from build123d import *

# Parameters (mm, degrees)
SKETCH1_W           = 10
SKETCH1_H           = 10
SKETCH1_R           = 2.25
BOSS_EXTRUDE1_DEPTH = 5
CUT_EXTRUDE1_START  = -1.75
CUT_EXTRUDE1_DEPTH  = 1.55
FILLET1_R           = 5


with BuildPart() as part:
    # Sketch1 → Boss-Extrude1 (new body)
    with BuildSketch(Plane(origin=(0, 0, 0), x_dir=(1, 0, 0), z_dir=(0, 1, 0))):
        Rectangle(SKETCH1_W, SKETCH1_H)
        with Locations(Location((0, 0, 0), (0, 0, 270))):
            Circle(SKETCH1_R, mode=Mode.SUBTRACT)
    extrude(amount=BOSS_EXTRUDE1_DEPTH)

    # Sketch2 → Cut-Extrude1 (cut)
    with BuildSketch(Plane(origin=(0, 5, 0), x_dir=(1, 0, 0), z_dir=(0, 1, 0)).offset(CUT_EXTRUDE1_START)):
        Polygon((-3, 5), (-5, 5), (-5, -5), (5, -5), (5, -3), (-3, -3), align=None)
    extrude(amount=-CUT_EXTRUDE1_DEPTH, mode=Mode.SUBTRACT)

    # Fillet1
    fillet1_edges = [part.edges().sort_by_distance(p)[0] for p in [
        (5, 2.5, -5),
    ]]
    fillet(fillet1_edges, radius=FILLET1_R)


solid = part.part
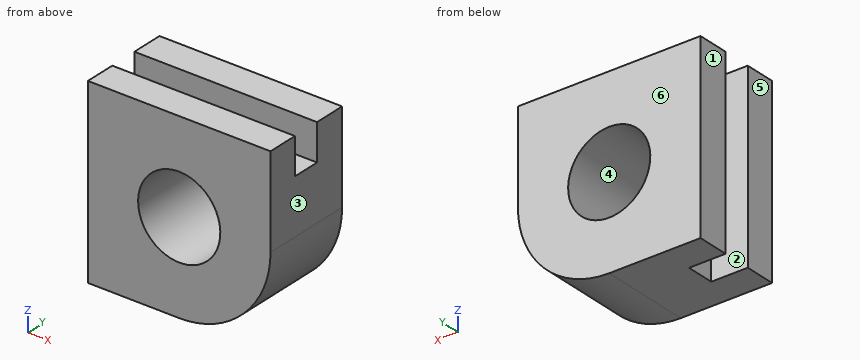
Can you work these out from the model? Positions are in its coordinate system, mm. Face numbers are marked on the shaded views. A direction names the side the tool comes from. Round coordinates to 2 decimals unless told otherwise and drop trailing zeros. Write each loop counter-clockwise with the first axis right and the second up, starting at its lowest first coordinate (ties: lowest second). Pieces come first, ordered by that corner, then holes. Notation, with made-up numbers: (34.5, 61) -> (80.5, 61) arc R24 cw to (80.5, 77) -> close; hole circle Ø11 at (80, -29). An arc over 180 degrees is marked (long way). Use one line per item in the form item = value. Start each with the question number.
Q1. Imagine slicing it at C-C (z = 2.75). Please give me the cut outline in (x, y), then the cut area to 3 significant figures.
Q2. Imagine slicing it at A-A (x = -4). Please give me the cut outline in (y, z), then the cut area to 3 significant figures.
Q3. Imagine slicing it at D-D (z = 0.5). Please give me the cut outline in (x, y).
Q4. If I drill on probe 1 along X at (y, z) = (3.05, 0); probe 2 along X at (y, z) = (0.95, 0); probe 3 along Y at (x, z) = (2.75, 3.5), over which ranges is the centre line in solid material (lowest first)? Write a range as [from, to].
Q5. We'd pull the mould along X, two halves only. Please class the marked faces 3, 4, 5 and 6: +X half, -X half, draft (parallel to the pull), parting line (faces both ways), or undercut.
Q6. I'm going to push flat-ended pins straight in: P1, Ø3, axis at y = 1.5, z = -3.5, coming from the +X side; P2, Ø2.5, axis at x = 0, z = 0, coming from the -Y side (3 decimals); P3, Ø3, axis at x = 1.5, z = -1.5, coming from the -Y side; P4, Ø1.5, axis at y = 4.5, z = -3.5, coming from the +X side. Where does each tip first touch, or does it pass through?
Q7. Imagine slicing it at B-B (y = 0.9). Please give me the cut outline in (x, z).
Q8. Which directions (+Z, -Z, +X, -X, +Y, -Y) give clear straight access to the entire face, cutting with the end or side of a thin tool? Please do the marked faces 1 and 2.
Worked out:
q1.outline = (-5, 0) -> (5, 0) -> (5, 5) -> (-5, 5) -> (-5, 3.25) -> (-3, 3.25) -> (-3, 1.7) -> (-5, 1.7) -> close
q1.area = 46.9 mm^2
q2.outline = (0, -5) -> (1.7, -5) -> (1.7, 5) -> (0, 5) -> close; (3.25, -5) -> (5, -5) -> (5, 5) -> (3.25, 5) -> close
q2.area = 34.5 mm^2
q3.outline = (-5, 0) -> (-2.19, 0) -> (-2.19, 5) -> (-5, 5) -> (-5, 3.25) -> (-3, 3.25) -> (-3, 1.7) -> (-5, 1.7) -> close; (2.19, 0) -> (5, 0) -> (5, 5) -> (2.19, 5) -> close
q4.probe_1 = [-3, -2.25], [2.25, 5]
q4.probe_2 = [-5, -2.25], [2.25, 5]
q4.probe_3 = [0, 1.7], [3.25, 5]
q5.face_3 = +X half
q5.face_4 = undercut
q5.face_5 = -X half
q5.face_6 = draft
q6.P1 = 4.58
q6.P2 = through
q6.P3 = 0
q6.P4 = 4.18
q7.outline = (-5, -5) -> (0, -5) arc R5 ccw to (5, 0) -> (5, 5) -> (-5, 5) -> close; hole circle Ø4.5 at (0, 0)
q8.face_1 = +Z, -Z, -X, +Y, -Y
q8.face_2 = +Z, -X
